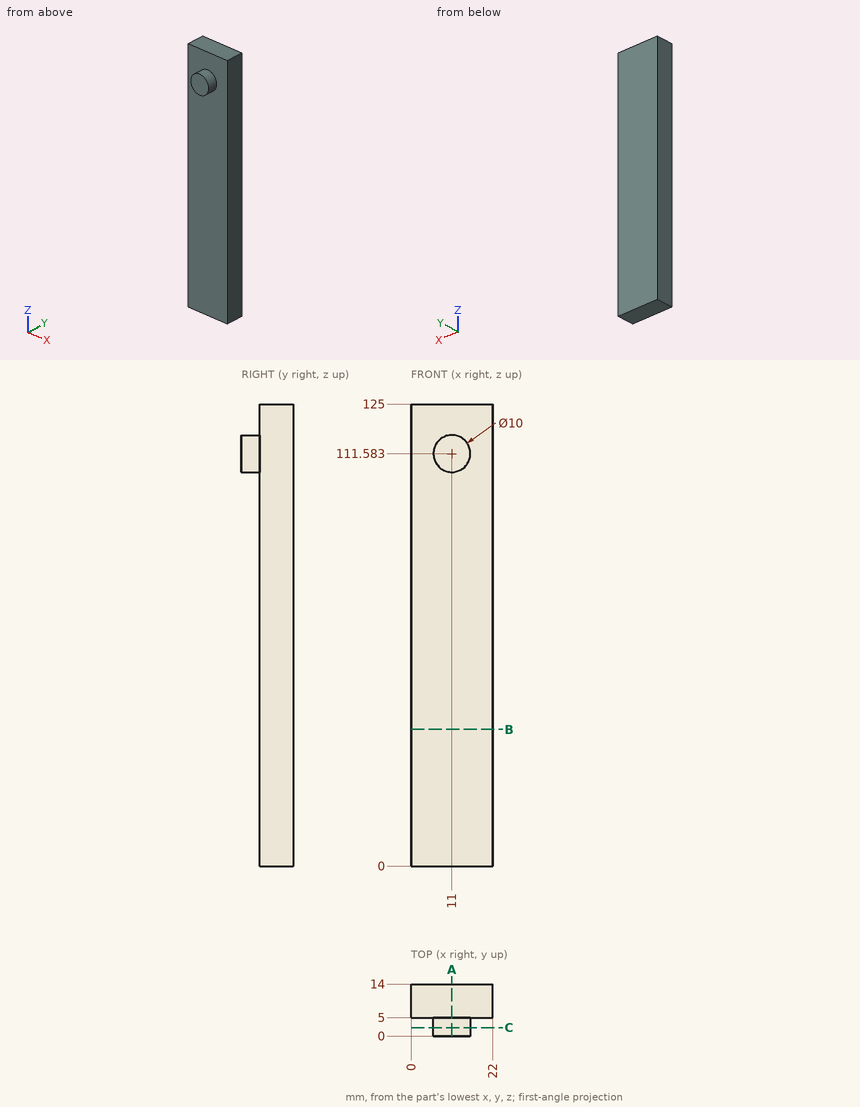
For this review, use the dimensioned drawing (mm, ordinates from the lowest corner) and the shaded views. Coordinates: 2 decimals unless noted, no trailing zeros. Loops run counter-clockwise (first coordinate to the right, second up) from the corner with the lowest first, then second, coordinate; pieces in that order, holes last. Notation, with made-up numbers: (13, 63) - (26, 63) arc R21 cw to (26, 76) - close; hole circle Ø10 at (56.25, 22.25). An arc over 180 degrees is marked (long way). Use CSV: the item, a comma, the result in double quotes. Start each with the question number.
1) Consider section C-C on y = 2.25. Write out the cut boundary in (x, z).
2) Consider section B-B on z = 37. Write out the cut boundary in (x, y).
3) For pin 1 Ø1.5 at (y, z) = (3, 81.5) entering from -X; pin 2 Ø4 at (x, z) = (17, 21) entering from -Y, all flat-tipped, find the tip position at first contact; note any pin that passes through.
4) Consider section A-A on x = 11. Write out the cut boundary in (y, z), then the cut area to 4 significant figures.
5) Wall thickness on L1, parallel to Y at x = 7.75, z = 90; L2, parallel to X at y = 2, z = 108.5; L3, parallel to Z at x = 8, y = 2.75: over which ranges is each line inside the solid? List them lowest first. Write a range as from..to.
Geometry says:
1,outline,"circle Ø10 at (11, 111.58)"
2,outline,"(0, 5) - (22, 5) - (22, 14) - (0, 14) - close"
3,pin 1,"through"
3,pin 2,"y = 5"
4,outline,"(0, 106.58) - (5, 106.58) - (5, 0) - (14, 0) - (14, 125) - (5, 125) - (5, 116.58) - (0, 116.58) - close"
4,area,"1,175 mm^2"
5,L1,"5..14"
5,L2,"7.06..14.94"
5,L3,"107.58..115.58"
